Could you check a few things on this model? Use its own coordinates, in mm. Give positions to 0.01 mm unless a question says otherwise; leave off trailing zeros. Order: outer loops, then holes, each group sorted by start corner. A loop starts at its lowest first (then second) coordinate and runs counter-clockwise, first axis right, second up. Notation, with made-up numbers: (28.25, -31.5) - (78.25, -31.5) arc R7 cw to (78.25, -18.5) - close; hole circle Ø5 at (34, 25.5). An arc over 180 degrees is marked (long way). Put each result on its own line as item: value.
from build123d import *

# Parameters (mm, degrees)
SKETCH2_R           = 2.5
BOSS_EXTRUDE1_DEPTH = 6


with BuildPart() as part:
    # Sketch2 → Boss-Extrude1 (new body)
    with BuildSketch(Plane(origin=(0, 0, 0), x_dir=(0, 0, -1), z_dir=(1, 0, 0))):
        Polygon((-64.527499051, -13), (-70.228832959, -3.125), (-70.228832959, 8.875), (-64.527499051, 18.75), (77.228832959, 18.75), (77.228832959, -13), align=None)
        Circle(SKETCH2_R, mode=Mode.SUBTRACT)
        with Locations((-25.039968051, 7)):
            Circle(SKETCH2_R, mode=Mode.SUBTRACT)
        with Locations((-52.228832959, 2.875)):
            Circle(SKETCH2_R, mode=Mode.SUBTRACT)
        with Locations((52.228832959, 2.875)):
            Circle(SKETCH2_R, mode=Mode.SUBTRACT)
        with Locations((25.039968051, 7)):
            Circle(SKETCH2_R, mode=Mode.SUBTRACT)
    extrude(amount=BOSS_EXTRUDE1_DEPTH)


solid = part.part
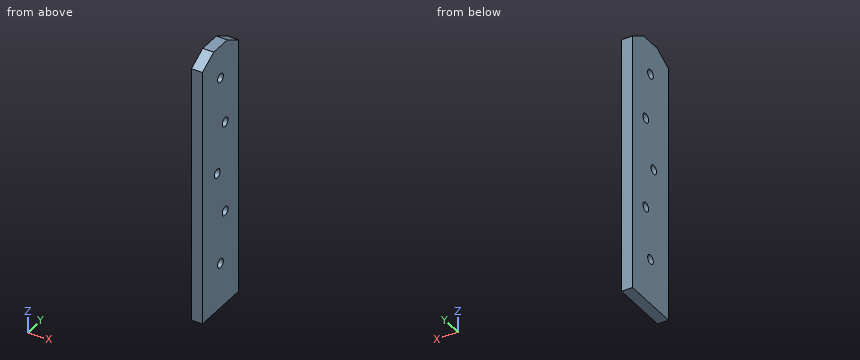
1) I'm going to push a flat-ended pin straight in: pin 1 (1.5 mm diameter, centred on x = 0.5, y = 13, fed in from +Z). Where does the tip first touch, or does it pass through?
Filled in:
pin 1: stops at z = 68.28
2) Suppose I cut it at A-A, the plane z = 0. List the corners of the cut face in (x, y) for me.
Filled in:
outline: (0, -13) - (6, -13) - (6, -2.5) - (0, -2.5) - close; (0, 2.5) - (6, 2.5) - (6, 18.75) - (0, 18.75) - close
3) Suppose I cut it at C-C, the plane x = 1.4. State how many separate pieces and enclosed holes the cut face has, and give its area (3 significant figures).
Filled in:
separate pieces: 1
enclosed holes: 5
area: 4,530 mm^2
4) If I drill on line 1 (Y direction, x = 4.1, z = 0); line 2 (Y direction, x = 0.95, z = -26); line 3 (Z direction, x = 3.25, y = -3.5), over which ranges is the centre line in solid material (lowest first)? Write a range as [from, to].
Filled in:
line 1: y = [-13, -2.5], [2.5, 18.75]
line 2: y = [-13, 4.69], [9.31, 18.75]
line 3: z = [-77.23, 70.01]
5) Suppose I cut it at B-B, the plane y = 7. List the corners of the cut face in (x, z) for me, and give its area (3 significant figures).
Filled in:
outline: (0, -77.23) - (6, -77.23) - (6, -27.54) - (0, -27.54) - close; (0, -22.54) - (6, -22.54) - (6, 22.54) - (0, 22.54) - close; (0, 27.54) - (6, 27.54) - (6, 70.23) - (0, 70.23) - close
area: 825 mm^2
